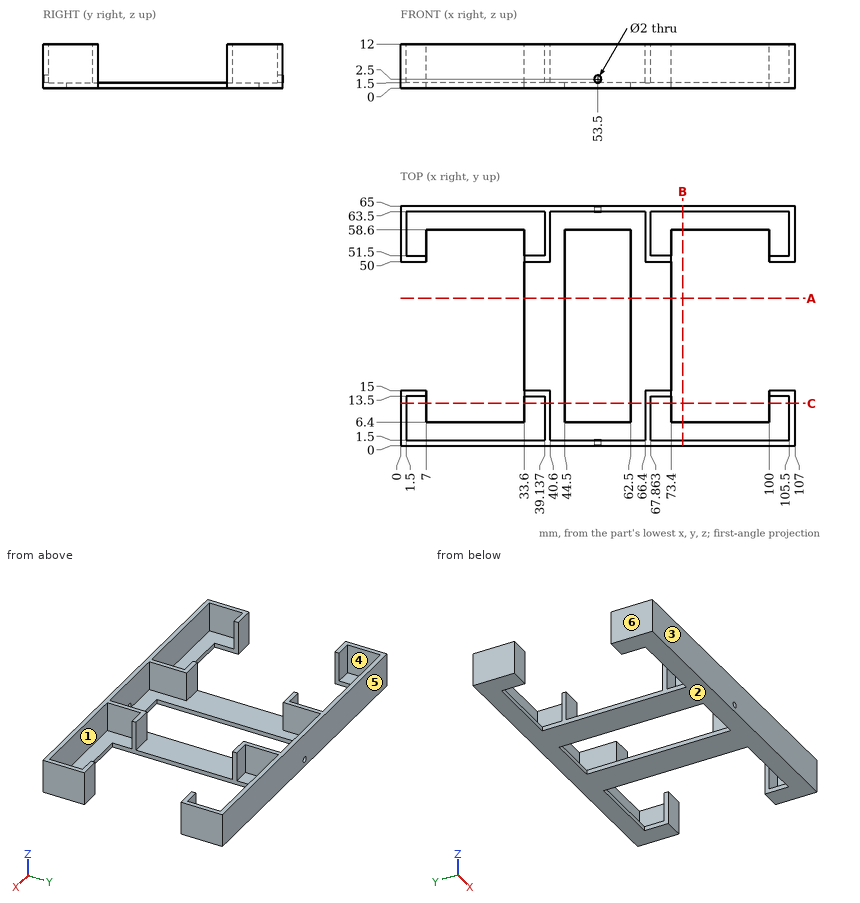
Geometry: see drawing. Coordinates: mm, zero at the bounding-box minimum. A direction names the side the tool comes from. Coordinates: 2 decimals unless noted, no trailing zeros. Order: outer loops, then holes, each group sorted by start corner. A loop starts at its lowest first (then second) coordinate and runs counter-clockwise, first axis right, second up. Notation, with made-up numbers: M 82.5,41 L 136.5,41 A9 cw 136.5,50 Z; hole C 22,71.5 d7. An arc over 180 degrees is marked long. Write item = value, one per line. Start each with the question number.
(1) Section A-A on y = 40. Output: boundary loops of the cut face in (x, z).
(2) Section C-C on y = 11.5. Output: boundary loops of the cut face in (x, z), and give its area (3 significant figures).
(3) Pull-direction query (Y, two-part tool) for the marked faces 3, 4, 5 and 6; classes: released by +Y, released by -Y, zero draft, split by the parting line, or undercut.
(4) First-contact query: P1, Ø5, axis at x = 94, z = 2, coming from the -Y side. Flat tip, straight axial feed; report the tip coordinate or a pass-through.
(5) Line query: line 1 along Y through (x, z) = (26.5, 9.75); line 2 along X through (y, z) = (64.4, 2.5); line 3 along Z through (x, y) = (53.5, 64.4). Output: solid intervals per line, ascending. Write a range as [from, to].
(6) Reachability of the marked faces 1 and 2 from +Z, -Z, +X, -X, +Y, -Y: full face, straight path, thin tool, end or side. Return the list, or none.
(7) Section B-B on x = 76.5. Output: boundary loops of the cut face in (y, z).
Result set:
q1.outline = M 33.6,0 L 44.5,0 L 44.5,1.5 L 33.6,1.5 Z; M 62.5,0 L 73.4,0 L 73.4,1.5 L 62.5,1.5 Z
q2.outline = M 0,0 L 7,0 L 7,1.5 L 1.5,1.5 L 1.5,12 L 0,12 Z; M 33.6,0 L 44.5,0 L 44.5,1.5 L 40.6,1.5 L 40.6,12 L 39.14,12 L 39.14,1.5 L 33.6,1.5 Z; M 62.5,0 L 73.4,0 L 73.4,1.5 L 67.86,1.5 L 67.86,12 L 66.4,12 L 66.4,1.5 L 62.5,1.5 Z; M 100,0 L 107,0 L 107,12 L 105.5,12 L 105.5,1.5 L 100,1.5 Z
q2.area = 116 mm²
q3.face_3 = released by -Y
q3.face_4 = undercut
q3.face_5 = released by +Y
q3.face_6 = zero draft
q4.P1 = 0
q5.line_1 = [0, 1.5], [63.5, 65]
q5.line_2 = [0, 52.5], [54.5, 107]
q5.line_3 = [0, 1.5], [3.5, 12]
q6.face_1 = +Z
q6.face_2 = -Z, +X, -X, +Y, -Y
q7.outline = M 0,0 L 6.4,0 L 6.4,1.5 L 1.5,1.5 L 1.5,12 L 0,12 Z; M 58.6,0 L 65,0 L 65,12 L 63.5,12 L 63.5,1.5 L 58.6,1.5 Z
